Work out the finished part from the listing and answer in its coordinate system (mm). Face numbers are marked on the shaded views. A direction names the side the tool comes from. Round coordinates to 2 decimals unless told otherwise and drop trailing zeros. Write each loop counter-clockwise with the first axis right and the second up, starting at its lowest first coordinate (ties: lowest second). Pieces come first, ordered by that corner, then holes. Notation, with made-up numbers: (-39, 75.25) - (8, 75.25) arc R34 ccw to (8, 113.25) - close; hole circle Ø1 at (-17.5, 41.5). An arc over 180 degrees is marked (long way). Answer as a JSON object with one key per item and string values.
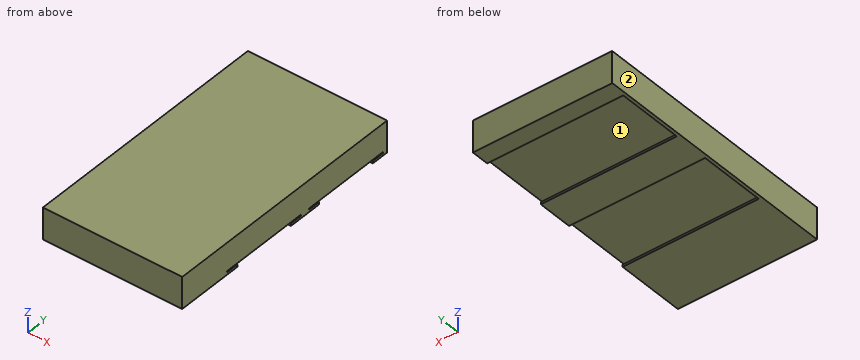
```python
from build123d import *

# Parameters (mm, degrees)
F0_W     = 88
F0_H     = 160
F1_DEPTH = 20
F3_DEPTH = 86


with BuildPart() as f1:
    # F0 (on Top) → F1 (new body)
    with BuildSketch(Plane.XY):
        with Locations((44, 80)):
            Rectangle(F0_W, F0_H)
    extrude(amount=F1_DEPTH)

    # F2 (on face) → F3 (cut)
    with BuildSketch(Plane.YZ.offset(88)):
        Polygon((107, 0), (149, 0), (149, 1.5), (157, 1.5), (157, 2.3), (99, 2.3), (99, 1.5), (107, 1.5), align=None)
        Polygon((93, 1.5), (93, 2.3), (35, 2.3), (35, 1.5), (43, 1.5), (43, 0), (85, 0), (85, 1.5), align=None)
    extrude(amount=-F3_DEPTH, mode=Mode.SUBTRACT)


solid = f1.part
```
Item 1: For the marked faces 1 and 2, determine the directions among +Z, -Z, +X, -X, +Y, -Y from which every point of the face is accessible in a straight line to the end or side of a thin tool.
Results found:
{"face 1": "+X", "face 2": "+Z, -Z, -X, +Y, -Y"}
Item 2: Consider line 1 along Z through (x, y) = (53.5, 101); line 2 along Z through (x, y) = (9, 133.5). Determine where each line is inside the solid, lowest interval first.
Results found:
{"line 1": "0 to 1.5, 2.3 to 20", "line 2": "2.3 to 20"}
Item 3: A cutting plane is placed at C-C (y = 77). Write down the section's boundary in (x, z), and give its area (3 significant figures).
Results found:
{"outline": "(0, 0) - (2, 0) - (2, 2.3) - (88, 2.3) - (88, 20) - (0, 20) - close", "area": "1,560 mm²"}
Item 4: A cutting plane is placed at A-A (y = 105). Write down the section's boundary in (x, z), and give its area (3 significant figures).
Results found:
{"outline": "(0, 0) - (88, 0) - (88, 1.5) - (2, 1.5) - (2, 2.3) - (88, 2.3) - (88, 20) - (0, 20) - close", "area": "1,690 mm²"}
Item 5: Each of these flat-tipped pins is pushed along its axis until it touches: P1, Ø1.2, axis at x = 41.5, z = 0.5, coming from the -Y side; P2, Ø12, axis at x = 32, y = 71, coming from the -Z side; P3, Ø2.5, axis at y = 141, z = 1, coming from the +X side. Where does it stop, or does it pass through?
Results found:
{"P1": "y = 0", "P2": "z = 2.3", "P3": "x = 2"}
Item 6: A cutting plane is placed at B-B (x = 48). Write down the section's boundary in (y, z), and give its area (3 significant figures).
Results found:
{"outline": "(0, 0) - (43, 0) - (43, 1.5) - (35, 1.5) - (35, 2.3) - (93, 2.3) - (93, 1.5) - (85, 1.5) - (85, 0) - (107, 0) - (107, 1.5) - (99, 1.5) - (99, 2.3) - (157, 2.3) - (157, 1.5) - (149, 1.5) - (149, 0) - (160, 0) - (160, 20) - (0, 20) - close", "area": "2,980 mm²"}
